The listing builds one solid part. Answer for the finished solid, in the listing's coordinates (mm). Face numbers are marked on the shaded views. A direction names the side the tool comes from. Give positions to 0.01 mm unless a question says otherwise; leave off trailing zeros. Order: outer loops, then holes, each group sorted by start corner. A loop starts at its lowest first (then second) coordinate and runs counter-clockwise, first axis right, second up. Notation, with made-up numbers: (-31.75, 44.5) - (-5.75, 44.5) arc R13 ccw to (-5.75, 56.5) - close; hole circle Ø9 at (14, 88). An arc over 180 degrees is marked (long way). Answer in a Markdown table with one row per item. Add a question column.
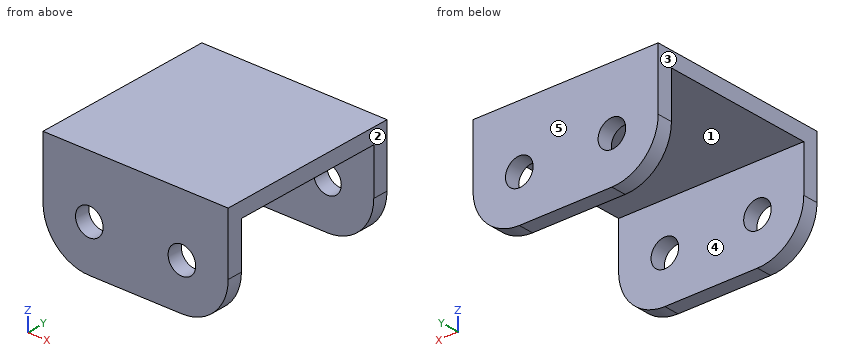
```python
from build123d import *

# Parameters (mm, degrees)
F0_R     = 2.25
F1_DEPTH = 15
F2_W     = 30.2
F2_H     = 30
F3_DEPTH = 2.5
F4_W     = 25
F4_H     = 7.55
F5_DEPTH = 30.201


with BuildPart() as f1:
    # F0 (on Front) → F1 (new body, symmetric)
    with BuildSketch(Plane.XZ):
        with BuildLine():
            ThreePointArc((-7.55, -7.55), (-2.211344, -5.338656), (0, 0))
            ThreePointArc((0, 0), (-2.211344, 5.338656), (-7.55, 7.55))
            ThreePointArc((-7.55, 7.55), (-12.888656, 5.338656), (-15.1, 0))
            ThreePointArc((-15.1, 0), (-12.888656, -5.338656), (-7.55, -7.55))
        make_face()
        with Locations((-7.55, 0)):
            Circle(F0_R, mode=Mode.SUBTRACT)
        with BuildLine():
            ThreePointArc((-15.1, 0), (-12.888656, 5.338656), (-7.55, 7.55))
            Line((-7.55, 7.55), (-15.1, 7.55))
            Line((-15.1, 7.55), (-15.1, 0))
        make_face()
        with BuildLine():
            ThreePointArc((-7.55, 7.55), (-2.211344, 5.338656), (0, 0))
            ThreePointArc((0, 0), (2.211344, 5.338656), (7.55, 7.55))
            Line((7.55, 7.55), (-7.55, 7.55))
        make_face()
        with BuildLine():
            Line((15.1, 7.55), (7.55, 7.55))
            ThreePointArc((7.55, 7.55), (12.888656, 5.338656), (15.1, 0))
            Line((15.1, 0), (15.1, 7.55))
        make_face()
        with BuildLine():
            ThreePointArc((7.55, -7.55), (2.211344, -5.338656), (0, 0))
            ThreePointArc((0, 0), (-2.211344, -5.338656), (-7.55, -7.55))
            Line((-7.55, -7.55), (7.55, -7.55))
        make_face()
        with BuildLine():
            ThreePointArc((7.55, 7.55), (2.211344, 5.338656), (0, 0))
            ThreePointArc((0, 0), (2.211344, -5.338656), (7.55, -7.55))
            ThreePointArc((7.55, -7.55), (12.888656, -5.338656), (15.1, 0))
            ThreePointArc((15.1, 0), (12.888656, 5.338656), (7.55, 7.55))
        make_face()
        with Locations((7.55, 0)):
            Circle(F0_R, mode=Mode.SUBTRACT)
    extrude(amount=F1_DEPTH, both=True)

    # F2 (on face) → F3 (join)
    with BuildSketch(Plane.XY.offset(7.55)):
        Rectangle(F2_W, F2_H)
    extrude(amount=F3_DEPTH)

    # F4 (on face) → F5 (cut, through all)
    with BuildSketch(Plane.YZ.offset(15.1)):
        with Locations((0, 3.775)):
            Rectangle(F4_W, F4_H)
        with Locations((0, -3.775)):
            Rectangle(F4_W, F4_H)
    extrude(amount=-F5_DEPTH, mode=Mode.SUBTRACT)


solid = f1.part
```
(1) The mould has two halves that part along Y. Classify the marked faces 3, 4 and 5: +Y half, -Y half, draft (parallel to the pull), parting line (faces both ways), or undercut.
(2) Find section A-A, the plane z = 3.25. Write down the section's boundary in (x, y), plus the area to 3 significant figures.
(3) Find section C-C, the plane y = -1.5. Write down the section's boundary in (x, z), plus the area to 3 significant figures.
(4) Each of these flat-tipped pins is pushed along its axis until it touches: P1, Ø5, axis at x = 7, y = 7, coming from the -Z side; P2, Ø3.5, axis at x = -7.55, z = 0, coming from the -Y side; P3, Ø4, axis at y = 12, z = -4.5, coming from the +X side. Where does it stop, or does it pass through?
(5) Find section B-B, the plane x = -1. Write down the section's boundary in (y, z).
(6) Straight lines are drawn through the part: line 1 (X direction, y = -13.6, z = 0); line 2 (Y direction, x = -3, z = 3.75); line 3 (Z direction, x = -7.55, y = 13.4). For each, find the intervals that lie inside material, in ascending order.
(7) For the marked faces 1 and 2, determine the directions among +Z, -Z, +X, -X, +Y, -Y from which every point of the face is accessible in a straight line to the end or side of a thin tool.
(8) Find section D-D, the plane z = -4.5. Write down the section's boundary in (x, y), plus the area to 3 significant figures.
Answer key:
| question | item | result |
|---|---|---|
| 1 | face 3 | draft |
| 1 | face 4 | undercut |
| 1 | face 5 | +Y half |
| 2 | outline | (-15.1, -15) - (15.1, -15) - (15.1, -12.5) - (-15.1, -12.5) - close; (-15.1, 12.5) - (15.1, 12.5) - (15.1, 15) - (-15.1, 15) - close |
| 2 | area | 151 mm² |
| 3 | outline | (-15.1, 7.55) - (15.1, 7.55) - (15.1, 10.05) - (-15.1, 10.05) - close |
| 3 | area | 75.5 mm² |
| 4 | P1 | z = 7.55 |
| 4 | P2 | through |
| 4 | P3 | x = 14.65 |
| 5 | outline | (-15, -7.55) - (-12.5, -7.55) - (-12.5, 7.55) - (12.5, 7.55) - (12.5, -7.55) - (15, -7.55) - (15, 10.05) - (-15, 10.05) - close |
| 6 | line 1 | -15.1 to -9.8, -5.3 to 5.3, 9.8 to 15.1 |
| 6 | line 2 | -15 to -12.5, 12.5 to 15 |
| 6 | line 3 | -7.55 to -2.25, 2.25 to 10.05 |
| 7 | face 1 | -Z, +X, -X |
| 7 | face 2 | +Z, -Z, +X, +Y, -Y |
| 8 | outline | (-13.61, -15) - (13.61, -15) - (13.61, -12.5) - (-13.61, -12.5) - close; (-13.61, 12.5) - (13.61, 12.5) - (13.61, 15) - (-13.61, 15) - close |
| 8 | area | 136 mm² |
